The model under review builds one solid part; all positions refer to its coordinate system, in mm. A direction names the side the tool comes from. Coordinates: 2 decimals unless noted, no trailing zeros. Order: outer loops, then holes, each group sorted by start corner. A loop starts at its lowest first (then second) coordinate and runs counter-clockwise, first axis right, second up. Notation, with made-up numbers: (72, 2.5) - (123, 2.5) arc R37 cw to (123, 38.5) - close; hole circle Ø2 at (56.25, 20). An arc over 180 degrees is marked (long way). Answer in a Markdown table with one row per item.
Autodesk Inventor part; units mm, degrees
ref_plane "YZ Plane" through (0, 0, 0) normal (1, 0, 0) x (0, 1, 0)
ref_plane "XZ Plane" through (0, 0, 0) normal (0, 1, 0) x (-1, 0, 0)
ref_plane "XY Plane" through (0, 0, 0) normal (0, 0, 1) x (1, 0, 0)
sketch "Sketch1" plane through (0, 0, 0) normal (1, 0, 0) x (0, 1, 0)
  line L0 (-44.45, 161.925) -> (-44.45, -161.925)
  line L1 (-44.45, -161.925) -> (44.45, -161.925)
  line L2 (44.45, -161.925) -> (44.45, 161.925)
  line L3 (44.45, 161.925) -> (-44.45, 161.925)
  line L4 (-44.45, 161.925) -> (44.45, -161.925) construction
  line L5 (-44.45, -161.925) -> (44.45, 161.925) construction
  point P0 (0, 0)
  dimension "d0" = 323.85
  dimension "d1" = 88.9
extrude "Extrusion1" add sketch "Sketch1" along normal mid plane 25.4
sketch "Sketch2" plane through (12.7, 0, 0) normal (1, 0, 0) x (0, 0, -1)
  line L0 (-161.925, -44.45) -> (161.925, -44.45)
  line L1 (-92.075, -44.45) -> (66.675, -44.45)
  line L2 (66.675, -44.45) -> (66.675, 0)
  line L3 (66.675, 0) -> (-92.075, 0)
  line L4 (-92.075, 0) -> (-92.075, -44.45)
  line L5 (-161.925, 44.45) -> (-161.925, -44.45)
  point P0 (0, 0)
  dimension "d4" = 158.75
  dimension "d5" = 44.45
  dimension "d6" = 69.85
extrude "Extrusion2" cut sketch "Sketch2" against normal through all
sketch "Sketch4" plane through (-12.7, -44.45, 161.925) normal (0, 0, 1) x (1, 0, 0)
  line L0 (7.9375, 0) -> (17.4625, 0)
  line L1 (17.4625, 0) -> (17.4625, 25.4)
  line L2 (17.4625, 25.4) -> (7.9375, 25.4)
  line L3 (7.9375, 25.4) -> (7.9375, 0)
  line L4 (25.4, 0) -> (0, 0)
  point P0 (12.7, 44.45)
  dimension "d11" = 4.7625
  dimension "d12" = 4.7625
  dimension "d13" = 25.4
extrude "Extrusion3" cut sketch "Sketch4" against normal through all
sketch "Sketch6" plane through (12.7, 0, 0) normal (1, 0, 0) x (0, 0, -1)
  point P0 (0, 0)
sketch "Sketch7" plane through (12.7, 0, 0) normal (1, 0, 0) x (0, 0, -1)
  line L0 (-161.925, 44.45) -> (-161.925, -44.45)
  line L1 (-161.925, -44.45) -> (-161.925, 44.45) construction
  line L2 (-161.925, -31.75) -> (161.925, -31.75) construction
  line L3 (161.925, 44.45) -> (161.925, -44.45) construction
  point P0 (0, 0)
  point P1 (-136.525, -31.75)
  point P2 (-111.125, -31.75)
  point P3 (117.475, -31.75)
  point P4 (142.875, -31.75)
  dimension "d16" = 12.7
  dimension "d17" = 25.4
  dimension "d18" = 25.4
  dimension "d19" = 279.4
  dimension "d20" = 25.4
hole "Hole1" at (12.7, -31.75, 136.525) at (12.7, -31.75, 111.125) at (12.7, -31.75, -117.475) at (12.7, -31.75, -142.875) direction (-1, 0, 0) diameter 6.7564 end through all
sketch "Sketch8" plane through (12.7, 0, 0) normal (1, 0, 0) x (0, 0, -1)
  line L0 (-161.925, 44.45) -> (-161.925, -44.45)
  line L1 (-161.925, 25.4) -> (-123.825, 25.4)
  line L2 (-123.825, 25.4) -> (-123.825, 44.45)
  line L3 (-123.825, 44.45) -> (-161.925, 44.45)
  line L4 (-161.925, 44.45) -> (-161.925, 25.4)
  line L5 (161.925, 44.45) -> (-161.925, 44.45)
  line L6 (161.925, 44.45) -> (161.925, -44.45)
  line L7 (161.925, 25.4) -> (123.825, 25.4)
  line L8 (123.825, 25.4) -> (123.825, 44.45)
  line L9 (123.825, 44.45) -> (161.925, 44.45)
  line L10 (161.925, 44.45) -> (161.925, 25.4)
  line L11 (-117.475, 44.45) -> (-79.375, 44.45)
  line L12 (-79.375, 44.45) -> (-79.375, 25.4)
  line L13 (-79.375, 25.4) -> (-117.475, 25.4)
  line L14 (-117.475, 25.4) -> (-117.475, 44.45)
  line L15 (104.775, 25.4) -> (66.675, 25.4)
  line L16 (66.675, 25.4) -> (66.675, 44.45)
  line L17 (66.675, 44.45) -> (104.775, 44.45)
  line L18 (104.775, 44.45) -> (104.775, 25.4)
  point P0 (0, 0)
  dimension "d28" = 38.1
  dimension "d29" = 19.05
  dimension "d30" = 6.35
  dimension "d31" = 146.05
extrude "Extrusion4" cut sketch "Sketch8" against normal through all
sketch "Sketch9" plane through (12.7, 25.4, 161.925) normal (0, 1, 0) x (1, 0, 0)
  line L0 (-17.4625, 0) -> (-7.9375, 0) construction
  line L1 (-12.7, 0) -> (-12.7, 323.226) construction
  line L2 (0, 0) -> (-25.4, 0) construction
  line L3 (0, 44.45) -> (-25.4, 44.45) construction
  line L4 (0, 228.6) -> (-25.4, 228.6) construction
  line L5 (0, 285.75) -> (-25.4, 285.75) construction
  point P0 (-12.7, 161.925)
  point P1 (-12.7, 19.05)
  point P2 (-12.7, 63.5)
  point P3 (-12.7, 247.65)
  point P4 (-12.7, 304.8)
  dimension "d34" = 19.05
  dimension "d35" = 19.05
  dimension "d36" = 19.05
  dimension "d37" = 19.05
hole "Hole2" at (0, 25.4, 142.875) at (0, 25.4, 98.425) at (0, 25.4, -85.725) at (0, 25.4, -142.875) direction (0, -1, 0) diameter 4.9784 depth 31.75 tip angle 118
equation "\"d0\" = RailSlideTotalLength"
equation "\"d1\" = RailSlideTotalHeight"
equation "\"d2\" = RailSlideTotalWidth"
equation "\"d4\" = WidthOfCutoutForTransmission"
equation "\"d5\" = heigthOfCutoutForTransmission"
equation "\"d6\" = distanceFromRearToStartOfTransmissionCutout"
equation "\"d7\" = RailSlideTotalWidth"
equation "\"d13\" = cutoutHeight"
equation "\"d14\" = RailSlideTotalWidth"
equation "\"d32\" = RailSlideTotalWidth"
equation "\"RailSlideTotalLength\" = 323.85"
equation "\"RailSlideTotalWidth\" = 25.4"
equation "\"RailSlideTotalHeight\" = 88.9"
equation "\"WidthOfCutoutForTransmission\" = 158.75"
equation "\"heigthOfCutoutForTransmission\" = 44.45"
equation "\"distanceFromRearToStartOfTransmissionCutout\" = 69.85"
equation "\"cutoutWidth\" = 9.525"
equation "\"cutoutHeight\" = 25.4"
properties part number "RailSlideLeftSide"
Item 1: Clearance check with flat-ended pins moving along their axes: pin 1 Ø6 at (x, z) = (-7, 53.5) entering from -Y; pin 2 Ø1.5 at (x, z) = (1, -96) entering from +Y; pin 3 Ø15 at (x, y) = (2, 34.5) entering from -Z (3 decimals). State where each tip first meets the part, or that it passes through.
Check values:
| item | result |
|---|---|
| pin 1 | y = 0 |
| pin 2 | y = 25.4 |
| pin 3 | z = -123.825 |
Item 2: We need section B-B, the plane x = -8.25. Write out the cut boundary in (y, z) (3 decimals), then the cut area to 3 significant figures.
Check values:
| item | result |
|---|---|
| outline | (-44.45, -161.925) - (25.4, -161.925) - (25.4, -123.825) - (44.45, -123.825) - (44.45, -104.775) - (25.4, -104.775) - (25.4, -66.675) - (44.45, -66.675) - (44.45, 79.375) - (25.4, 79.375) - (25.4, 117.475) - (44.45, 117.475) - (44.45, 123.825) - (25.4, 123.825) - (25.4, 161.925) - (-44.45, 161.925) - (-44.45, 92.075) - (0, 92.075) - (0, -66.675) - (-44.45, -66.675) - close; hole circle Ø6.756 at (-31.75, -142.875); hole circle Ø6.756 at (-31.75, -117.475); hole circle Ø6.756 at (-31.75, 111.125); hole circle Ø6.756 at (-31.75, 136.525) |
| area | 18,700 mm^2 |
Item 3: To check wall thickness, follow line 1 (Z direction, x = -10.75, y = -31.75) (3 decimals); line 2 (Z direction, x = 0, y = -3.5) (3 decimals); line 3 (Z direction, x = 0, y = 10) (3 decimals). State the ranges of each line that lie inside material, in increasing order. Write a range as from..to.
Check values:
| item | result |
|---|---|
| line 1 | -161.925..-146.253, -139.497..-120.853, -114.097..-66.675, 92.075..107.747, 114.503..133.147, 139.903..161.925 |
| line 2 | -161.925..-145.364, -140.386..-88.214, -83.236..-66.675, 92.075..95.936, 100.914..140.386, 145.364..161.925 |
| line 3 | -161.925..-145.364, -140.386..-88.214, -83.236..95.936, 100.914..140.386, 145.364..161.925 |
Item 4: Tool access review of faces 1 (the face through (0, 35, -66.675)), 2 (the face through (0, -18, -66.675)), 3 (the face through (0, -19.05, -114)): name each direction out of +Z, -Z, +X, -X, +Y, -Y from which nothing blocks a thin tool from reaching the whole face with its end or side.
Check values:
| item | result |
|---|---|
| face 1 | +X, -X, +Y |
| face 2 | +X, -X, -Y |
| face 3 | +Z, -Z, -Y |
Item 5: Mouldability with a two-part tool opening along X and no side actions: class faces 4 (the face through (8.676, -29.694, 139.206)), 5 (the face through (12.7, 9, 2)), 6 (the face through (-4.762, -32, 127)) as +X half, -X half, draft (parallel to the pull), parting line (faces both ways), or undercut.
Check values:
| item | result |
|---|---|
| face 4 | draft |
| face 5 | +X half |
| face 6 | undercut |
Item 6: We need section D-D, the plane z = -131. Write out the cut boundary in (x, y).
Check values:
| item | result |
|---|---|
| outline | (-12.7, -44.45) - (-4.76, -44.45) - (-4.76, -19.05) - (4.76, -19.05) - (4.76, -44.45) - (12.7, -44.45) - (12.7, 25.4) - (-12.7, 25.4) - close |
Item 7: We need section C-C, the plane y = -39. Write out the cut boundary in (x, z) (1 decimal).
Check values:
| item | result |
|---|---|
| outline | (-12.7, -161.9) - (-4.8, -161.9) - (-4.8, -66.7) - (-12.7, -66.7) - close; (-12.7, 92.1) - (-4.8, 92.1) - (-4.8, 161.9) - (-12.7, 161.9) - close; (4.8, -161.9) - (12.7, -161.9) - (12.7, -66.7) - (4.8, -66.7) - close; (4.8, 92.1) - (12.7, 92.1) - (12.7, 161.9) - (4.8, 161.9) - close |
Item 8: We need section A-A, the plane y = 36.5. Write out the cut boundary in (x, z) (3 decimals), then the cut area to 3 significant figures.
Check values:
| item | result |
|---|---|
| outline | (-12.7, -123.825) - (12.7, -123.825) - (12.7, -104.775) - (-12.7, -104.775) - close; (-12.7, -66.675) - (12.7, -66.675) - (12.7, 79.375) - (-12.7, 79.375) - close; (-12.7, 117.475) - (12.7, 117.475) - (12.7, 123.825) - (-12.7, 123.825) - close |
| area | 4,350 mm^2 |
